The model under review builds one solid part; all positions refer to its coordinate system, in mm. A direction names the side the tool comes from. Give positions to 0.01 mm unless a question says otherwise; leave off trailing zeros. Loops run counter-clockwise (first coordinate to the right, second up) from the corner with the lowest first, then second, coordinate; pieces in that order, holes last. Notation, with made-up numbers: M 43,71 L 76,71 A16 ccw 76,79 Z; hole C -26.75,-9.75 d2. An arc over 180 degrees is marked long. Put each result on its own line as item: value. Start each with the question number.
from build123d import *

# Parameters (mm, degrees)
ESQUISSE1_R        = 40
ESQUISSE1_R_2      = 25
BOSS_EXTRU_1_DEPTH = 25
BOSS_EXTRU_2_START = -10
ESQUISSE4_R        = 6
ESQUISSE4_R_2      = 25
BOSS_EXTRU_2_DEPTH = 10
CONG_1_R           = 5


with BuildPart() as part:
    # Esquisse1 → Boss.-Extru.1 (new body)
    with BuildSketch(Plane.XY):
        Circle(ESQUISSE1_R)
        Circle(ESQUISSE1_R_2, mode=Mode.SUBTRACT)
    extrude(amount=BOSS_EXTRU_1_DEPTH)

    # Esquisse4 → Boss.-Extru.2 (add)
    with BuildSketch(Plane.XY.offset(25).offset(BOSS_EXTRU_2_START)):
        with BuildLine():
            Line((41, 46), (-41, 46))
            ThreePointArc((-41, 46), (-44.535533906, 44.535533906), (-46, 41))
            Line((-46, 41), (-46, -41))
            ThreePointArc((-46, -41), (-44.535533906, -44.535533906), (-41, -46))
            Line((-41, -46), (41, -46))
            ThreePointArc((41, -46), (44.535533906, -44.535533906), (46, -41))
            Line((46, -41), (46, 41))
            ThreePointArc((46, 41), (44.535533906, 44.535533906), (41, 46))
        make_face()
        with Locations((-36, 36)):
            Circle(ESQUISSE4_R, mode=Mode.SUBTRACT)
        with Locations((-36, -36)):
            Circle(ESQUISSE4_R, mode=Mode.SUBTRACT)
        with Locations(Location((36, -36, 0), (0, 0, 180))):
            Circle(ESQUISSE4_R, mode=Mode.SUBTRACT)
        with Locations(Location((36, 36, 0), (0, 0, 180))):
            Circle(ESQUISSE4_R, mode=Mode.SUBTRACT)
        Circle(ESQUISSE4_R_2, mode=Mode.SUBTRACT)
    extrude(amount=BOSS_EXTRU_2_DEPTH)

    # Congé1
    # the kernel refuses this fillet: 5 mm, written as the material it adds along each edge
    with BuildSketch(Plane(origin=(0, 0, 15), x_dir=(1, 0, 0), z_dir=(0, 1, 0))) as cong_1_piece_1_section:
        with BuildLine():
            CenterArc((40 + CONG_1_R, CONG_1_R), CONG_1_R, 180, 90)
            Line((40 + CONG_1_R, 0), (40, 0))
            Line((40, 0), (40, CONG_1_R))
        make_face()
    cong_1_piece_1 = revolve(axis=Axis((0, 0, 15), (0, 0, -1)), mode=Mode.PRIVATE)
    cong_1_piece_1 = cong_1_piece_1 - Plane(origin=(36, 36, 13.61437319), x_dir=(-1, 0, 0), z_dir=(0, 0, -1)) * Cylinder(6, 180, mode=Mode.PRIVATE)
    cong_1_piece_1 = cong_1_piece_1 - Plane(origin=(-36, 36, 13.61437319), x_dir=(1, 0, 0), z_dir=(0, 0, -1)) * Cylinder(6, 180, mode=Mode.PRIVATE)
    cong_1_piece_1 = cong_1_piece_1 - Plane(origin=(36, -36, 13.61437319), x_dir=(-1, 0, 0), z_dir=(0, 0, -1)) * Cylinder(6, 180, mode=Mode.PRIVATE)
    cong_1_piece_1 = cong_1_piece_1 - Plane(origin=(-36, -36, 13.61437319), x_dir=(1, 0, 0), z_dir=(0, 0, -1)) * Cylinder(6, 180, mode=Mode.PRIVATE)
    add(cong_1_piece_1)


solid = part.part
(1) For faces 1 (the cylindrical face through (40.76, 32.35, 19.93)), 2 (the cylindrical face through (-8.67, -39.05, 4.93)), list the 3-axis set-ups (+Z, -Z, +X, -X, +Y, -Y) from which the entire face can be reached by the end or side of a thin tool; tool diameter is ignored.
(2) To check wall thickness, follow L1, parallel to X at y = -36, z = 19.75; L2, parallel to Y at x = 0.5, z = 7.25 (3 decimals). State the ranges of each line that lie inside material, in increasing order. Write a range as [from, to].
(3) Insertion check: pin 1 (2 mm diameter, centred on y = -27, z = 9.5, fed in from +X); pin 2 (2 mm diameter, centred on x = 9, z = 5, fed in from -Y); pin 3 (1 mm diameter, centred on x = 14.5, z = 3.5, fed in from +Y). Each pin has a flat end and moves straight along its axis. Give the tip position at first contact, or say it passes through.
(4) We need section D-D, the plane z = 13. Write out the cut boundary in (x, y), plus the area to 3 significant figures.
(5) Draft analysis for pull direction X (two halves, no side actions). For faces 3 (the cylindrical face through (23.846, 7.509, 12.325)), 4 (the cylindrical face through (-44, 45, 20)), 5 (the flat face through (17.22, 18.34, 0)), 6 (the flat face through (46, -1, 20)), state which applies: +X half, -X half, draft (parallel to the pull), parting line (faces both ways), or undercut.
(6) We need section A-A, the plane y = 0. Write out the cut boundary in (x, z), plus the area to 3 significant figures.
(7) We need section B-B, the plane z = 23. Write out the cut boundary in (x, y).
Check sheet entries:
1. face 1: +Z, -Z
1. face 2: -Z
2. L1: x = [-46, -42], [-30, 30], [42, 46]
2. L2: y = [-39.997, -24.995], [24.995, 39.997]
3. pin 1: stops at x = 30.4
3. pin 2: stops at y = -39.19
3. pin 3: stops at y = 37.47
4. outline: C 0,0 d82; hole C 0,0 d50
4. area: 3,320 mm²
5. face 3: undercut
5. face 4: -X half
5. face 5: draft
5. face 6: +X half
6. outline: M -46,15 L -45,15 A5 cw -40,10 L -40,0 L -25,0 L -25,25 L -46,25 Z; M 25,0 L 40,0 L 40,10 A5 cw 45,15 L 46,15 L 46,25 L 25,25 Z
6. area: 881 mm²
7. outline: M -46,-41 A5 ccw -41,-46 L 41,-46 A5 ccw 46,-41 L 46,41 A5 ccw 41,46 L -41,46 A5 ccw -46,41 Z; hole C -36,-36 d12; hole C -36,36 d12; hole C 0,0 d50; hole C 36,-36 d12; hole C 36,36 d12
